Could you check a few things on this model? Use its own coordinates, in mm. Give positions to 0.01 mm unless a question says otherwise; leave off trailing zeros. Loops run counter-clockwise (first coordinate to the right, second up) from the corner with the lowest first, then second, coordinate; pieces in that order, holes last. Notation, with made-up numbers: (-4.75, 35.25) -> (52.25, 35.25) arc R22 cw to (52.25, 56.25) -> close; hole circle Ø7 at (-19.5, 32.25). An arc over 180 degrees is marked (long way). Write item = value, one per line. Start each with the question number.
1) I want a section at C-C (z = -42). List the corners of the cut face in (x, y) for me.
2) I want a section at D-D (x = 28). List the corners of the cut face in (y, z) for me.
3) I'm going to push a flat-ended pin straight in: pin 1 Ø6 at (x, z) = (108, 39) entering from -Y. Where does the tip first touch, or does it pass through?
4) I want a section at A-A (y = -42.5). List the corners of the cut face in (x, z) for me.
5) I want a section at B-B (x = 110). List the corners of the cut face in (y, z) for me.
6) I need wall thicknesses on probe 1 along Y at (x, z) = (20.5, 46); probe 2 along X at (y, z) = (-48, 9); probe 3 along X at (y, z) = (-44, -1). Which ranges of each line are inside material? Lowest first, please. Write a range as from..to.
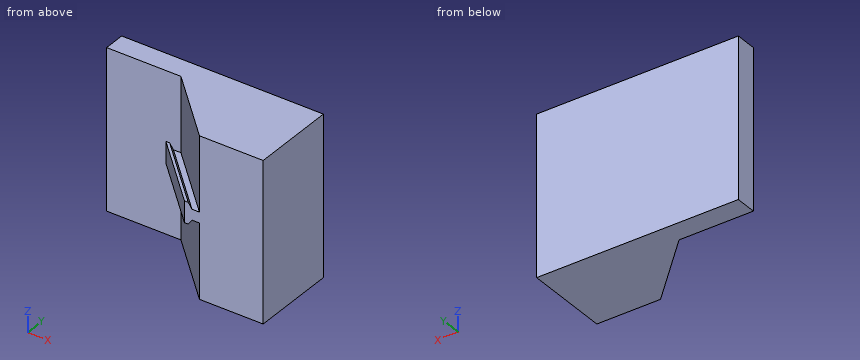
from build123d import *

# Parameters (mm, degrees)
EXTRUDE_1_DEPTH          = 75
EXTRUDE_2_REACH          = 181.652
EXTRUDE_3_DEPTH          = 150
EXTRUDE_4_DEPTH          = 14.142135624
CUT_EXTRUDE_2_DEPTH      = 267.643072547
CUT_EXTRUDE_2_DEPTH_BACK = 267.643072547
SKETCH_5_W               = 110.242252028
SKETCH_5_H               = 36.038971429
CUT_EXTRUDE_3_DEPTH      = 265.95282599
CUT_EXTRUDE_3_DEPTH_BACK = 265.95282599
SKETCH_6_W               = 40.565596645
SKETCH_6_H               = 160.869683045


with BuildPart() as part:
    # 草图1 → 凸台-拉伸1 (new, symmetric)
    with BuildSketch(Plane.XY):
        Polygon((0, 0), (70, 0), (120, -50), (210, -50), (210, 20), (0, 20), align=None)
    extrude(amount=EXTRUDE_1_DEPTH, both=True)

    # 凸台-拉伸2: up to this plane
    extrude_2_end = Plane(origin=(0, 0, 75), z_dir=(0, 1, 0))
    # 草图2 → 凸台-拉伸2 (add, up to the surface)
    with BuildSketch(Plane(origin=(85, -85, 0), x_dir=(0, 0, -1), z_dir=(-0.7071067811865562, 0.7071067811865388, 0)), mode=Mode.PRIVATE) as extrude_2_sk1:
        Polygon((5, -44.497474683), (10, -41.997474683), (10, -39.497474683), (-10, -39.497474683), (-10, -41.997474683), (-5, -44.497474683), (-5, -54.497474683), (5, -54.497474683), align=None)
    extrude_2_tool1 = split(extrude(extrude_2_sk1.sketch, amount=EXTRUDE_2_REACH, mode=Mode.PRIVATE), bisect_by=extrude_2_end, keep=Keep.BOTH, mode=Mode.PRIVATE)
    add(extrude_2_tool1.solids().sort_by_distance((117.446559, -52.553441, 0))[0])

    # 草图4 → 凸台-拉伸3 (add)
    with BuildSketch(Plane.XY.offset(75)):
        Polygon((120, -50), (130, -60), (210, -60), (210, -50), align=None)
    extrude(amount=-EXTRUDE_3_DEPTH)

    # 草图2<2> → 凸台-拉伸4 (add)
    with BuildSketch(Plane(origin=(85, -85, 0), x_dir=(0, 0, -1), z_dir=(-0.7071067811865562, 0.7071067811865388, 0))):
        Polygon((5, -44.497474683), (10, -41.997474683), (10, -39.497474683), (-10, -39.497474683), (-10, -41.997474683), (-5, -44.497474683), (-5, -54.497474683), (5, -54.497474683), align=None)
    extrude(amount=-EXTRUDE_4_DEPTH)

    # 草图5 → 切除-拉伸2 (cut, two sides: drawn at the far end of the back side and taken through both)
    with BuildSketch(Plane(origin=(0, 0, -75), x_dir=(-1, 0, 0), z_dir=(0, 0, -1)).offset(-CUT_EXTRUDE_2_DEPTH_BACK)):
        with Locations((-132.449509919, -78.019485715)):
            Rectangle(SKETCH_5_W, SKETCH_5_H)
    extrude(amount=CUT_EXTRUDE_2_DEPTH + CUT_EXTRUDE_2_DEPTH_BACK, mode=Mode.SUBTRACT)

    # 草图6 → 切除-拉伸3 (cut, two sides: drawn at the far end of the back side and taken through both)
    with BuildSketch(Plane.XY.offset(75).offset(-CUT_EXTRUDE_3_DEPTH_BACK)):
        with Locations((210.282798323, -41.689599735)):
            Rectangle(SKETCH_6_W, SKETCH_6_H)
    extrude(amount=CUT_EXTRUDE_3_DEPTH + CUT_EXTRUDE_3_DEPTH_BACK, mode=Mode.SUBTRACT)


solid = part.part
Answer list:
q1.outline = (0, 0) -> (70, 0) -> (130, -60) -> (190, -60) -> (190, 20) -> (0, 20) -> close
q2.outline = (0, -75) -> (20, -75) -> (20, 75) -> (0, 75) -> close
q3.pin_1 = -41
q4.outline = (98.36, -10) -> (101.89, -10) -> (105.43, -5) -> (112.5, -5) -> (112.5, -75) -> (190, -75) -> (190, 75) -> (112.5, 75) -> (112.5, 5) -> (105.43, 5) -> (101.89, 10) -> (98.36, 10) -> close
q5.outline = (-54.14, -10) -> (-50.61, -10) -> (-47.07, -5) -> (-40, -5) -> (-40, -75) -> (20, -75) -> (20, 75) -> (-40, 75) -> (-40, 5) -> (-47.07, 5) -> (-50.61, 10) -> (-54.14, 10) -> close
q6.probe_1 = 0..20
q6.probe_2 = 103.86..108.1, 118..190
q6.probe_3 = 99.86..190
